Build history of the part. All positions in model axes, mm. Give positions to 0.01 mm unless a question says otherwise; leave off trailing zeros. Order: outer loops, then holes, each group sorted by start corner. A loop starts at its lowest first (then second) coordinate and runs counter-clockwise, first axis right, second up. Notation, with made-up numbers: (57.5, 68.25) -> (80.5, 68.25) arc R16 cw to (80.5, 73.25) -> close; hole circle Ø4 at (35.5, -14.75). An arc over 180 degrees is marked (long way). One line per item, written item: value. Start each with the question number.
(1) Saw through at B-B on x = 36.83. Give the cut face in (y, z) (1 decimal).
(2) Saw through at A-A on x = 0. Give the cut face in (y, z) (1 decimal), plus the area to 3 significant figures.
(3) Probe line 1 (X direction, y = 0.1, z = -19.5); line 2 (Z direction, x = 0, y = 0.6) (3 decimals); line 3 (Z direction, x = 31.75, y = 1) (3 decimals). List the from-to ranges inside material, lowest first.
```python
from build123d import *

# Parameters (mm, degrees)
SKETCH1_W             = 78.74
SKETCH1_H             = 44.45
BOSS_EXTRUDE1_DEPTH   = 1.5875
F_4_CLEARANCE_HOLE1_D = 3.2639
F_4_CLEARANCE_HOLE2_D = 3.2639


with BuildPart() as part:
    # Sketch1 → Boss-Extrude1 (new body)
    with BuildSketch(Plane(origin=(0, 0, 0), x_dir=(1, 0, 0), z_dir=(0, 1, 0))):
        Rectangle(SKETCH1_W, SKETCH1_H)
    extrude(amount=BOSS_EXTRUDE1_DEPTH)

    # #4 Clearance Hole1 (through all)
    with Locations(Plane(origin=(0, 1.5875, 0), x_dir=(1, 0, 0), z_dir=(0, 1, 0))):
        with Locations((-36.83, 19.685), (36.83, 19.685), (31.75, -19.685), (-31.75, -19.685)):
            Hole(F_4_CLEARANCE_HOLE1_D / 2)

    # #4 Clearance Hole2 (through all)
    with Locations(Plane(origin=(0, 1.5875, 0), x_dir=(1, 0, 0), z_dir=(0, 1, 0))):
        with Locations((0, 8.762995682), (0, -15.113004318)):
            Hole(F_4_CLEARANCE_HOLE2_D / 2)


solid = part.part
```
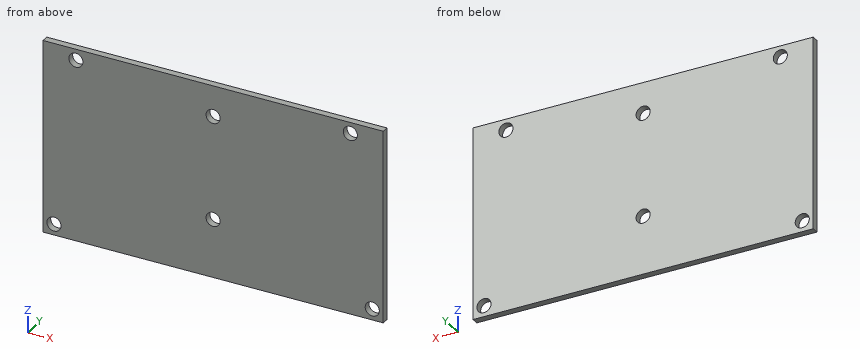
Results below:
1. outline: (0, -22.2) -> (1.6, -22.2) -> (1.6, -21.3) -> (0, -21.3) -> close; (0, -18.1) -> (1.6, -18.1) -> (1.6, 22.2) -> (0, 22.2) -> close
2. outline: (0, -22.2) -> (1.6, -22.2) -> (1.6, -10.4) -> (0, -10.4) -> close; (0, -7.1) -> (1.6, -7.1) -> (1.6, 13.5) -> (0, 13.5) -> close; (0, 16.7) -> (1.6, 16.7) -> (1.6, 22.2) -> (0, 22.2) -> close
2. area: 60.2 mm²
3. line 1: x = -39.37 to -38.45, -35.21 to 35.21, 38.45 to 39.37
3. line 2: z = -22.225 to -10.395, -7.131 to 13.481, 16.745 to 22.225
3. line 3: z = -22.225 to 18.053, 21.317 to 22.225
